from build123d import *

# Parameters (mm, degrees)
FILLET1_R              = 2
MOVE_FACE1_BY          = 2
MOVE_FACE4_BY          = 1.8
MOVE_START             = 1.2
MOVE_FACE3_OUTLINE_R   = 4.05
MOVE_FACE3_OUTLINE_R_2 = 4
MOVE_FACE3_DEPTH       = 4.8
CHAMFER1_SIZE          = 2


# Read off the part's stored shape, not the designer's step: Move Face3
with BuildPart() as part:
    # Sketch2 → Revolve1 (revolve)
    with BuildSketch(Plane.XY, mode=Mode.PRIVATE) as revolve1_sk:
        Polygon((2.6, 0), (2.6, 3), (4, 3), (4, 6), (9.671572875, 6), (9.671572875, 5.5), (7.171572875, 3), (9.671572875, 0.5), (9.671572875, 0), align=None)
    revolve(revolve1_sk.sketch.rotate(Axis((0, 0, 0), (0, 1, 0)), 90), axis=Axis((0, 0, 0), (0, 1, 0)))

    # Fillet1
    fillet1_edges = [part.edges().sort_by_distance(p)[0] for p in [
        (0, 3, 7.171572875),
    ]]
    fillet(fillet1_edges, radius=FILLET1_R)

    # Move Face1: a face moved outward by 2.0
    extrude(part.faces().sort_by_distance((4.835786438, 0, 0))[0], amount=MOVE_FACE1_BY, dir=(0, -1, 0))

    # Move Face4: a face moved inward by 1.8
    extrude(part.faces().sort_by_distance((3.2, 3, 0))[0], amount=MOVE_FACE4_BY, dir=(0, -1, 0), mode=Mode.SUBTRACT)

    # Move Face3 outline → Move Face3 (cut)
    with BuildSketch(Plane(origin=(0, 0, 0), x_dir=(1, 0, 0), z_dir=(0, 1, 0)).offset(MOVE_START)):
        Circle(MOVE_FACE3_OUTLINE_R)
        Circle(MOVE_FACE3_OUTLINE_R_2, mode=Mode.SUBTRACT)
    extrude(amount=MOVE_FACE3_DEPTH, mode=Mode.SUBTRACT)

    # Chamfer1
    chamfer1_edges = [part.edges().sort_by_distance(p)[0] for p in [
        (0, -2, 9.671572875),
    ]]
    chamfer(chamfer1_edges, length=CHAMFER1_SIZE - 0.0001)  # a hair under: the kernel refuses the full size


solid = part.part
For this review, take the finished solid that the model builds, in its own axes (mm). A direction names the side the tool comes from. Coordinates: 2 decimals unless noted, no trailing zeros. Loops run counter-clockwise (first coordinate to the right, second up) from the corner with the lowest first, then second, coordinate; pieces in that order, holes last. Notation, with made-up numbers: (40, -21.5) - (71, -21.5) arc R24 cw to (71, 6.5) - close; hole circle Ø5 at (24, 10.25). An arc over 180 degrees is marked (long way). Use a Markdown table: item, result. Add a question column.
Item 1: Tool access review of faces 1 (the face through (-0.1, 6, 4.2)), 2 (the face through (0, 1.2, 3)): name each direction out of +Z, -Z, +X, -X, +Y, -Y from which nothing blocks a thin tool from reaching the whole face with its end or side.
Item 2: Mouldability with a two-part tool opening along X and no side actions: class faces 3 (the face through (0, -2, -3)), 4 (the face through (8.58, 0.25, -4.46)), 5 (the face through (-2.578, -0.378, 0.338)) as pulls with the +X half, pulls with the -X half, needs draft (parallel to the pull), parting line crosses it, or undercut.
Item 3: Insertion check: pin 1 Ø4 at (x, z) = (0.5, -1.5) entering from +Y. The pin has a flat end and moves straight along its axis. Give the tip position at first contact, or say it passes through.
Item 4: We need section A-A (y = -1.25). Give the boundary of the cut face in (x, z), and give its area (3 significant figures).
Item 5: We need section B-B (y = 5.25). Give the boundary of the cut face in (x, z).
Item 6: For line 1 (X direction, y = 0.25, z = 0); line 2 (Y direction, x = -1.75, z = 3.25); line 3 (Z direction, x = -0.75, y = 2.75), list the stretches that pass through material, from the lowest coordinate up.
Results list:
| question | item | result |
|---|---|---|
| 1 | face 1 | +Z, -Z, +X, -X, +Y |
| 1 | face 2 | +Y |
| 2 | face 3 | needs draft |
| 2 | face 4 | parting line crosses it |
| 2 | face 5 | undercut |
| 3 | pin 1 | stops at y = 1.2 |
| 4 | outline | circle Ø16.84 at (0, 0); hole circle Ø5.2 at (0, 0) |
| 4 | area | 202 mm^2 |
| 5 | outline | circle Ø18.84 at (0, 0); hole circle Ø8.1 at (0, 0) |
| 6 | line 1 | x = -9.67 to -2.6, 2.6 to 9.67 |
| 6 | line 2 | y = -2 to 1.2 |
| 6 | line 3 | z = -7.98 to -3.98, 3.98 to 7.98 |
